Input: part model. Units: mm. Frame: model coordinates. Give positions to 0.01 mm unless a question says otherwise; leave off trailing zeros. Loops run counter-clockwise (first coordinate to the right, second up) from the corner with the lowest first, then second, coordinate; pieces in that order, holes last. Notation, with made-up numbers: (-3.5, -11) - (25.5, -11) arc R12 ccw to (25.5, -7) - close; hole circle Ø11 at (-3, 88.25). An arc over 180 degrees is marked (long way). Answer as a JSON object with one key per item and string values.
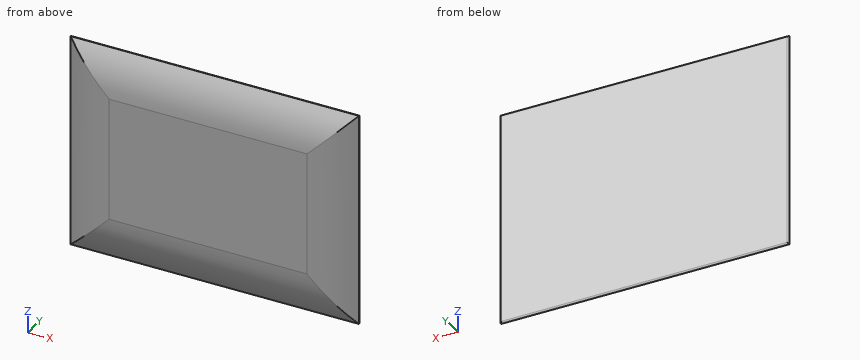
from build123d import *

# Parameters (mm, degrees)
SKETCH1_W           = 182
SKETCH1_H           = 135
BOSS_EXTRUDE1_DEPTH = 9
FILLET4_R           = 1
FILLET5_R           = 55


with BuildPart() as part:
    # Sketch1 → Boss-Extrude1 (new body)
    with BuildSketch(Plane(origin=(0, 0, 0), x_dir=(1, 0, 0), z_dir=(0, 1, 0))):
        Rectangle(SKETCH1_W, SKETCH1_H)
    extrude(amount=BOSS_EXTRUDE1_DEPTH)

    # Fillet4
    fillet4_edges = [part.edges().sort_by_distance(p)[0] for p in [
        (-91, 9, 0),
        (0, 9, 67.5),
        (91, 9, 0),
        (0, 9, -67.5),
    ]]
    fillet(fillet4_edges, radius=FILLET4_R)

    # Fillet5
    # the kernel refuses this fillet: 55 mm, written as the material it takes off along each edge
    with BuildSketch(Plane(origin=(162.414284285, 0, -67.5), x_dir=(0, 0, 1), z_dir=(-1, 0, 0))) as fillet5_piece_1:
        with BuildLine():
            CenterArc((28.565713714, 55), FILLET5_R, 238.709554786, 31.290445214)
            Line((0, 8), (0, 0))
            Line((0, 0), (28.565713714, 0))
        make_face()
    extrude(amount=324.828568571, mode=Mode.SUBTRACT)
    with BuildSketch(Plane(origin=(-91, 0, -138.914284285), x_dir=(0, 1, 0), z_dir=(0, 0, 1))) as fillet5_piece_2:
        with BuildLine():
            CenterArc((55, -28.565713714), FILLET5_R, 148.709554786, 31.290445214)
            Line((0, -28.565713714), (0, 0))
            Line((0, 0), (8, 0))
        make_face()
    extrude(amount=277.828568571, mode=Mode.SUBTRACT)
    with BuildSketch(Plane(origin=(-162.414284285, 0, 67.5), x_dir=(0, 1, 0), z_dir=(1, 0, 0))) as fillet5_piece_3:
        with BuildLine():
            CenterArc((55, -28.565713714), FILLET5_R, 148.709554786, 31.290445214)
            Line((0, -28.565713714), (0, 0))
            Line((0, 0), (8, 0))
        make_face()
    extrude(amount=324.828568571, mode=Mode.SUBTRACT)
    with BuildSketch(Plane(origin=(91, 0, 138.914284285), x_dir=(-1, 0, 0), z_dir=(0, 0, -1))) as fillet5_piece_4:
        with BuildLine():
            CenterArc((28.565713714, 55), FILLET5_R, 238.709554786, 31.290445214)
            Line((0, 8), (0, 0))
            Line((0, 0), (28.565713714, 0))
        make_face()
    extrude(amount=277.828568571, mode=Mode.SUBTRACT)


solid = part.part
Item 1: Cut plane A-A (x = -54). Return loops of the section in (y, z).
Geometry check:
{"outline": "(0, -38.93) arc R55 ccw to (8, -67.5) arc R1 ccw to (9, -66.5) - (9, 66.5) arc R1 ccw to (8, 67.5) arc R55 ccw to (0, 38.93) - close"}
Item 2: Cut plane B-B (z = 22). Return loops of the section in (x, y).
Geometry check:
{"outline": "(-91, 8) arc R55 ccw to (-62.43, 0) - (62.43, 0) arc R55 ccw to (91, 8) arc R1 ccw to (90, 9) - (-90, 9) arc R1 ccw to start"}
Item 3: Contact query for flat-ended pins moving along their axis: P1, Ø1.5, axis at x = 51.5, y = 4.5, coming from the -Z side; P2, Ø4, axis at y = 5, z = -36.5, coming from the +X side; P3, Ø5, axis at y = 2.5, z = -5, coming from the +X side. Output: stop coordinate, or through.
Geometry check:
{"P1": "stops at z = -62.39", "P2": "stops at x = 89.29", "P3": "stops at x = 85.35"}
Item 4: Cut plane C-C (y = 2.25). Return loops of the section in (x, z).
Geometry check:
{"outline": "(-78, -54.5) - (78, -54.5) - (78, 54.5) - (-78, 54.5) - close"}
Item 5: Material intervals for line 1 (Y direction, x = -77.5, z = -3.5); line 2 (Y direction, x = -47, z = -39); line 3 (Z direction, x = 31, y = 6.75), sorted ascending. Write a range as [from, to].
Geometry check:
{"line 1": "y = [2.1, 9]", "line 2": "y = [0, 9]", "line 3": "z = [-65.33, 65.33]"}
